Can you work these out from the drawing? Everything is in mm from the part's minimum corner. Round coordinates to 2 decimals unless told otherwise and drop trailing zeros. Loops run counter-clockwise (first coordinate to the right, second up) from the corner with the lowest first, then second, coordinate; pieces in that order, holes last. Notation, with made-up numbers: (70, 7) -> (78, 7) arc R9 ccw to (78, 11) -> close; hole circle Ø4 at (5.5, 57). An arc over 180 degrees is marked (long way). One line per item, written item: value.
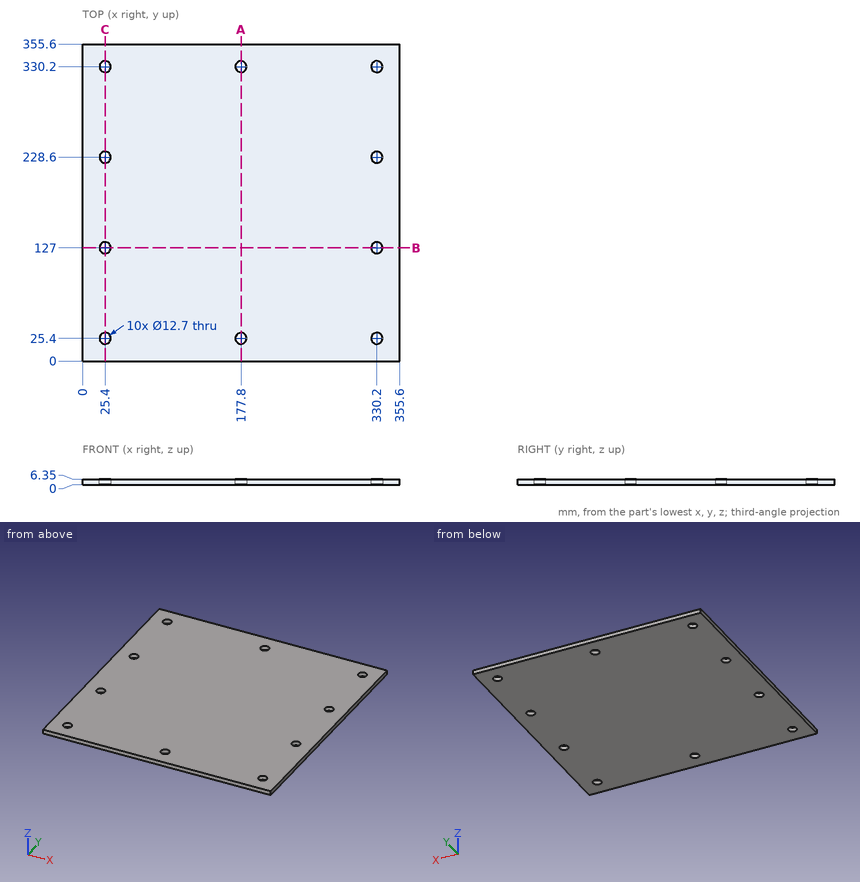
Item 1: If we section it at A-A on x = 177.8: List the corners of the cut face in (y, z) for me, plus the area to 3 significant figures.
Output:
outline: (0, 0) -> (19.05, 0) -> (19.05, 6.35) -> (0, 6.35) -> close; (31.75, 0) -> (323.85, 0) -> (323.85, 6.35) -> (31.75, 6.35) -> close; (336.55, 0) -> (355.6, 0) -> (355.6, 6.35) -> (336.55, 6.35) -> close
area: 2,100 mm²
Item 2: I need wall thicknesses on line 1 (Y direction, x = 25.4, z = 2); line 2 (Y direction, x = 177.8, z = 1.75); line 3 (Y direction, x = 335, z = 5.5). Which ranges of each line are inside material? Lowest first, please. Write a range as from..to.
Output:
line 1: y = 0..19.05, 31.75..120.65, 133.35..222.25, 234.95..323.85, 336.55..355.6
line 2: y = 0..19.05, 31.75..323.85, 336.55..355.6
line 3: y = 0..21.24, 29.56..122.84, 131.16..224.44, 232.76..326.04, 334.36..355.6
Item 3: If we section it at C-C on x = 25.4: List the corners of the cut face in (y, z) for me, plus the area to 3 significant figures.
Output:
outline: (0, 0) -> (19.05, 0) -> (19.05, 6.35) -> (0, 6.35) -> close; (31.75, 0) -> (120.65, 0) -> (120.65, 6.35) -> (31.75, 6.35) -> close; (133.35, 0) -> (222.25, 0) -> (222.25, 6.35) -> (133.35, 6.35) -> close; (234.95, 0) -> (323.85, 0) -> (323.85, 6.35) -> (234.95, 6.35) -> close; (336.55, 0) -> (355.6, 0) -> (355.6, 6.35) -> (336.55, 6.35) -> close
area: 1,940 mm²
